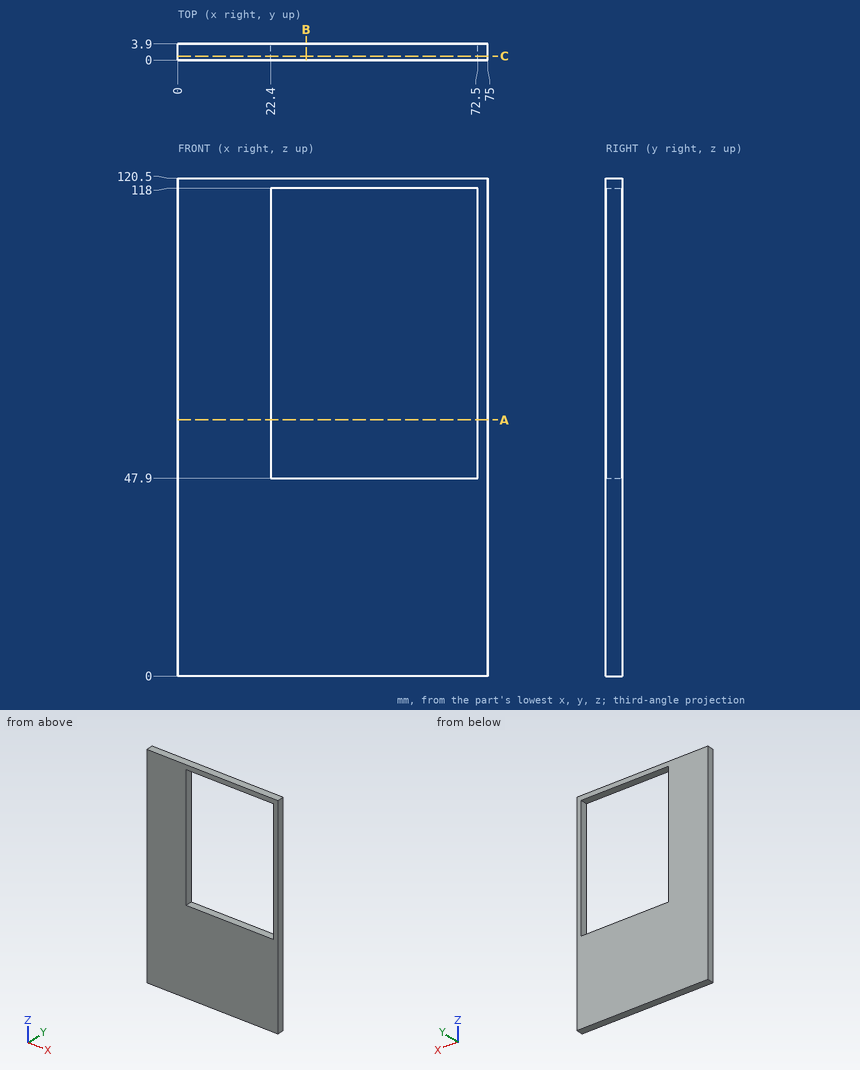
Input: dimensioned drawing with shaded views. Units: mm. Origin: part minimum x, y, z. Give positions to 0.01 mm unless a question says otherwise; leave off trailing zeros. Order: outer loops, then holes, each group sorted by start corner. A loop starts at its lowest first (then second) coordinate and runs counter-clockwise, first axis right, second up. Notation, with made-up numbers: (23.25, 60) -> (79.25, 60) arc R30 ccw to (79.25, 96) -> close; hole circle Ø11 at (-17.75, -19). An arc over 180 degrees is marked (long way). Answer as a JSON object with one key per item and string values.
Q1. Section B-B (x = 31). Output: boundary loops of the cut face in (y, z).
Entries:
{"outline": "(0, 0) -> (3.9, 0) -> (3.9, 47.9) -> (0, 47.9) -> close; (0, 118) -> (3.9, 118) -> (3.9, 120.5) -> (0, 120.5) -> close"}
Q2. Material intervals for probe 1 along Z at (x, y) = (30, 2.4); probe 2 along X at (y, z) = (1.05, 69), sorted ascending.
Entries:
{"probe 1": "z = 0 to 47.9, 118 to 120.5", "probe 2": "x = 0 to 22.4, 72.5 to 75"}
Q3. Section A-A (z = 62). Output: boundary loops of the cut face in (x, y), plus the area to 3 significant figures.
Entries:
{"outline": "(0, 0) -> (22.4, 0) -> (22.4, 3.9) -> (0, 3.9) -> close; (72.5, 0) -> (75, 0) -> (75, 3.9) -> (72.5, 3.9) -> close", "area": "97.1 mm^2"}
Q4. Section C-C (y = 0.95). Output: boundary loops of the cut face in (x, z), plus the area to 3 significant figures.
Entries:
{"outline": "(0, 0) -> (75, 0) -> (75, 120.5) -> (0, 120.5) -> close; hole (22.4, 47.9) -> (72.5, 47.9) -> (72.5, 118) -> (22.4, 118) -> close", "area": "5,530 mm^2"}
Q5. First-contact query: pin 1 (2 mm diameter, centred on y = 3, z = 78.5, fed in from -X). Flat tip, straight axial feed; report the tip coordinate or a pass-through.
Entries:
{"pin 1": "stops at x = 0"}
